from build123d import *

# Parameters (mm, degrees)
SKETCH1_W           = 4.82
SKETCH1_H           = 4.14
SKETCH2_R           = 2.5
BOSS_EXTRUDE1_DEPTH = 20
CUT_EXTRUDE1_DEPTH  = 2.5
CHAMFER1_SIZE       = 0.4905
FILLET1_R           = 0.414


with BuildPart() as part:
    # Sketch1 → Revolve1 (revolve)
    with BuildSketch(Plane(origin=(0, 0, 0), x_dir=(-1, 0, 0), z_dir=(0, 0, -1)), mode=Mode.PRIVATE) as revolve1_sk:
        with Locations((2.41, 2.07)):
            Rectangle(SKETCH1_W, SKETCH1_H)
    revolve(revolve1_sk.sketch.rotate(Axis((0, 0, 0), (-1, 0, 0)), 270), axis=Axis((0, 0, 0), (-1, 0, 0)))

    # Sketch2 → Boss-Extrude1 (add)
    with BuildSketch(Plane(origin=(0, 0, 0), x_dir=(0, 0, -1), z_dir=(1, 0, 0))):
        Circle(SKETCH2_R)
    extrude(amount=BOSS_EXTRUDE1_DEPTH)

    # Sketch3 → Cut-Extrude1 (cut)
    with BuildSketch(Plane.ZY.offset(4.82)):
        Polygon((-2, -1.154700538), (0, -2.309401077), (2, -1.154700538), (2, 1.154700538), (0, 2.309401077), (-2, 1.154700538), align=None)
    extrude(amount=-CUT_EXTRUDE1_DEPTH, mode=Mode.SUBTRACT)

    # Chamfer1
    chamfer1_edges = [part.edges().sort_by_distance(p)[0] for p in [
        (20, 0, 2.5),
    ]]
    chamfer(chamfer1_edges, length=CHAMFER1_SIZE)

    # Fillet1
    fillet1_edges = [part.edges().sort_by_distance(p)[0] for p in [
        (-4.82, 0, -4.14),
    ]]
    fillet(fillet1_edges, radius=FILLET1_R)


solid = part.part
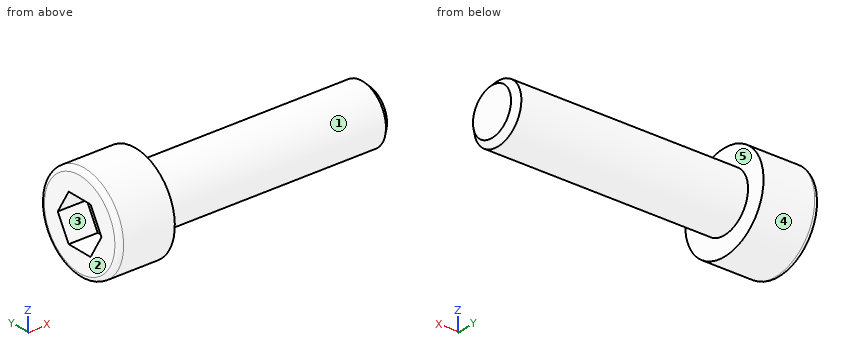
Build history of the part. All positions in model axes, mm. Face numbers are marked on the shaded views. A direction names the side the tool comes from. Round coordinates to 2 decimals unless told otherwise and drop trailing zeros. Write each loop counter-clockwise with the first axis right and the second up, starting at its lowest first coordinate (ties: lowest second). Pieces come first, ordered by that corner, then holes. Notation, with made-up numbers: M 53,-24 L 81,-24 A18 ccw 81,3 Z; hole C 79,20.25 d5. An arc over 180 degrees is marked long. Use CSV: the item, a comma, the result in double quotes.
1. Saw through at C-C (x = -0.5). Give the cut face in (y, z), plus the area to 3 significant figures.
Reply:
outline,"C 0,0 d8.28"
area,"53.8 mm²"
2. Two-plate mould, pull along Y, no slides. Class the marked faces 1, 2 and 3: +Y half, -Y half, draft (parallel to the pull), parting line (faces both ways), or undercut.
Reply:
face 1,"parting line"
face 2,"draft"
face 3,"undercut"
3. Flat gauge pins, fed straight in: pin 1 (4 mm diameter, centred on x = 5, y = -1.5, fed in from -Z); pin 2 (2 mm diameter, centred on x = 4.5, z = 1, fed in from +Y); pin 3 (1.5 mm diameter, centred on x = 11.5, z = -2, fed in from +Y). Where does each tip first touch, or does it go through?
Reply:
pin 1,"stops at z = -2.5"
pin 2,"stops at y = 2.5"
pin 3,"stops at y = 2.17"
4. Wall check: probe 1 along X at (y, z) = (0.75, -3.5); probe 2 along Z at (x, y) = (15.25, 1.5); probe 3 along Z at (x, y) = (-3, 1). Give the ranges that are in metal, low to high. Write a range as from..to.
Reply:
probe 1,"x = -4.82..0"
probe 2,"z = -2..2"
probe 3,"z = -4.02..-2, 2..4.02"
5. Tool access for the marked faces 4 and 5: list every direction of +Z, -Z, +X, -X, +Y, -Y with a clear straight run to the whole face (end or side of a thin tool).
Reply:
face 4,"+X, -X"
face 5,"+X"
6. Saw through at A-A (y = 0). Give the cut face in (x, z).
Reply:
outline,"M -4.82,-3.73 A0.41 ccw -4.41,-4.14 L 0,-4.14 L 0,-2.5 L 19.51,-2.5 L 20,-2.01 L 20,2.01 L 19.51,2.5 L 0,2.5 L 0,4.14 L -4.41,4.14 A0.41 ccw -4.82,3.73 L -4.82,2 L -2.32,2 L -2.32,-2 L -4.82,-2 Z"
7. Saw through at B-B (x = 4). Give the cut face in (y, z), plus the area to 3 significant figures.
Reply:
outline,"C 0,0 d5"
area,"19.6 mm²"
